from build123d import *

# Parameters (mm, degrees)
F0_W     = 196
F0_H     = 120
F0_R     = 2
F1_DEPTH = 4
F2_R     = 1.75
F3_DEPTH = 6


with BuildPart() as f1:
    # F0 (on Top) → F1 (new body)
    with BuildSketch(Plane.XY):
        with Locations((22.739595, 0)):
            Rectangle(F0_W, F0_H)
        with Locations((14.739595, 0)):
            Circle(F0_R, mode=Mode.SUBTRACT)
        with Locations((30.739595, 0)):
            Circle(F0_R, mode=Mode.SUBTRACT)
    extrude(amount=F1_DEPTH)

    # F2 (on face) → F3 (join)
    with BuildSketch(Plane.XY.offset(4)):
        with Locations((-66.260405, -51)):
            Circle(F2_R)
        with Locations((22.989595, -51)):
            Circle(F2_R)
        with Locations((111.739595, -42)):
            Circle(F2_R)
        with Locations((111.739595, 42)):
            Circle(F2_R)
        with Locations((-52.260405, 51)):
            Circle(F2_R)
        with Locations((-66.260405, 0)):
            Circle(F2_R)
        with Locations((97.739595, 51)):
            Circle(F2_R)
        with Locations((27.739595, 51)):
            Circle(F2_R)
        with Locations((111.739595, 0)):
            Circle(F2_R)
    extrude(amount=F3_DEPTH)


solid = f1.part
Could you check a few things on this model? Use its own coordinates, in mm. A direction names the side the tool comes from. Coordinates: 2 decimals unless noted, no trailing zeros. Loops run counter-clockwise (first coordinate to the right, second up) from the corner with the lowest first, then second, coordinate; pieces in that order, holes last.
1. We'd pull the mould along X, two halves only. Please class faces 1 (the face through (21.601, -52.065, 6.958)), 2 (the face through (32.587, -0.766, 1.972)), 3 (the face through (112, -42, 10)), 4 (the face through (-75.26, -1, 2)): released by +X, released by -X, zero draft, split by the parting line, or undercut.
2. Imagine slicing it at A-A (z = 8.5). Give the number of separate pieces and of enclosed holes in the cut face, and give its area (3 significant figures).
3. Imagine slicing it at B-B (y = -13). Please give me the cut outline in (x, z), and give its area (3 significant figures).
4. For P1, Ø2, axis at x = -2.5, y = 30.5, coming from the -Z side; P2, Ø1, axis at x = 9, y = 3.5, coming from the +Z side, each with a flat end and sliding along its axis, tell me the tip position at first contact or that it passes through.
5. Imagine slicing it at C-C (x = -20.5). Please give me the cut outline in (y, z).
6. I need wall thicknesses on L1, parallel to Z at x = -18, y = 28; L2, parallel to Y at x = -52.5, z = 4.5; L3, parallel to X at y = -43, z = 8.75. Which ranges of each line are inside material? Lowest first, please.
7. For faces 5 (the face through (112, 0, 10)), 6 (the face through (-64.644, -51.67, 6.958)), which set-ups out of +Z, -Z, +X, -X, +Y, -Y let a thin tool reach every point of the face, with its end or its side?
Computed values:
1. face 1: undercut
1. face 2: undercut
1. face 3: zero draft
1. face 4: released by -X
2. separate pieces: 9
2. enclosed holes: 0
2. area: 86.6 mm2
3. outline: (-75.26, 0) - (120.74, 0) - (120.74, 4) - (-75.26, 4) - close
3. area: 784 mm2
4. P1: stops at z = 0
4. P2: stops at z = 4
5. outline: (-60, 0) - (60, 0) - (60, 4) - (-60, 4) - close
6. L1: z = 0 to 4
6. L2: y = 49.27 to 52.73
6. L3: x = 110.3 to 113.18
7. face 5: +Z, +X, -X, +Y, -Y
7. face 6: +Z
